Part model, mm, in its own coordinate system. Face numbers are marked on the shaded views. A direction names the side the tool comes from. Coordinates: 2 decimals unless noted, no trailing zeros. Loops run counter-clockwise (first coordinate to the right, second up) from the corner with the lowest first, then second, coordinate; pieces in that order, holes last. Notation, with made-up numbers: (-29, 59) -> (-6, 59) arc R28 ccw to (-6, 87) -> close; hole circle Ø11 at (75, 55). An arc over 180 degrees is marked (long way). One line per item, written item: value. Start each with the question number.
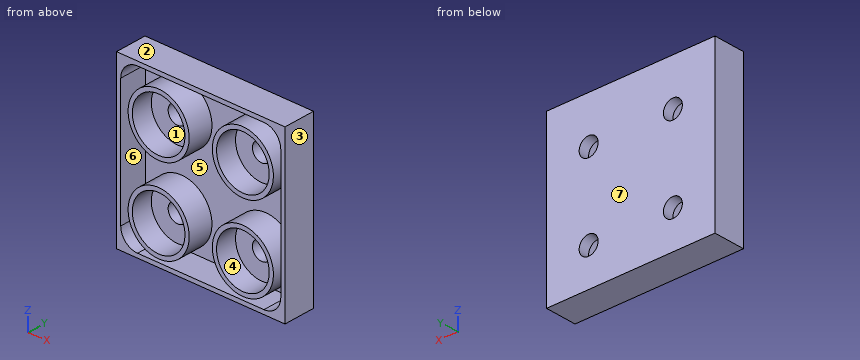
from build123d import *

# Parameters (mm, degrees)
CROQUIS1_W              = 40
CROQUIS1_H              = 40
CROQUIS1_R              = 2.25
SALIENTE_EXTRUIR1_DEPTH = 7.5
CROQUIS2_R              = 6.25
CORTAR_EXTRUIR1_DEPTH   = 5
VACIADO1_T              = -1
REDONDEO1_R             = 4


with BuildPart() as part:
    # Croquis1 → Saliente-Extruir1 (new body)
    with BuildSketch(Plane(origin=(0, 0, 0), x_dir=(1, 0, 0), z_dir=(0, 1, 0))):
        Rectangle(CROQUIS1_W, CROQUIS1_H)
        with Locations(Location((-10, -9, 0), (0, 0, 270))):
            Circle(CROQUIS1_R, mode=Mode.SUBTRACT)
        with Locations(Location((10, -9, 0), (0, 0, 270))):
            Circle(CROQUIS1_R, mode=Mode.SUBTRACT)
        with Locations(Location((10, 11, 0), (0, 0, 270))):
            Circle(CROQUIS1_R, mode=Mode.SUBTRACT)
        with Locations(Location((-10, 11, 0), (0, 0, 270))):
            Circle(CROQUIS1_R, mode=Mode.SUBTRACT)
    extrude(amount=SALIENTE_EXTRUIR1_DEPTH)

    # Croquis2 → Cortar-Extruir1 (cut)
    with BuildSketch(Plane.XZ):
        with Locations(Location((-10, 9, 0), (0, 0, 270))):
            Circle(CROQUIS2_R)
        with Locations(Location((10, 9, 0), (0, 0, 270))):
            Circle(CROQUIS2_R)
        with Locations(Location((-10, -11, 0), (0, 0, 270))):
            Circle(CROQUIS2_R)
        with Locations(Location((10, -11, 0), (0, 0, 270))):
            Circle(CROQUIS2_R)
    extrude(amount=-CORTAR_EXTRUIR1_DEPTH, mode=Mode.SUBTRACT)

    # Vaciado1
    vaciado1_openings = [part.faces().sort_by_distance(p)[0] for p in [
        (0, 0, 0.442577116),
    ]]
    offset(amount=VACIADO1_T, openings=vaciado1_openings, kind=Kind.INTERSECTION)

    # Redondeo1
    redondeo1_edges = [part.edges().sort_by_distance(p)[0] for p in [
        (-19, 3.25, -19),
        (19, 3.25, -19),
        (19, 3.25, 19),
        (-19, 3.25, 19),
    ]]
    fillet(redondeo1_edges, radius=REDONDEO1_R)


solid = part.part
1) Tool access for the marked faces 5, 6 and 7: list every direction of +Z, -Z, +X, -X, +Y, -Y with a clear straight run to the whole face (end or side of a thin tool).
2) Slice it at A-A (y = 3.5). State how many separate pieces and enclosed holes the cut face has, then the cut area to 3 significant figures.
3) Pull direction Z, two halves, no side cores. Call the marked faces 1, 2, 3 and 4: +Z half, -Z half, draft (parallel to the pull), parting line (faces both ways), or undercut.
4) Probe line 1 (X direction, y = 1.35, z = 9); line 2 (X direction, y = 3.5, z = -1); line 3 (X direction, y = 6.2, z = 9). List the from-to ranges inside material, lowest first. Write a range as from..to.
5) Slice it at B-B (z = -2.5). Give the cut face in (x, y), then the cut area to 3 significant figures.
6) Pin check, flat tips, straight feed: pin 1 Ø12 at (x, z) = (6, -15) entering from -Y; pin 2 Ø7 at (x, z) = (10, -11) entering from -Y. Stop position of each tip, or through.
Check sheet entries:
1. face 5: none
1. face 6: -Y
1. face 7: +Z, -Z, +X, -X, +Y
2. separate pieces: 5
2. enclosed holes: 5
2. area: 339 mm^2
3. face 1: undercut
3. face 2: +Z half
3. face 3: draft
3. face 4: undercut
4. line 1: x = -20..-19, -17.25..-16.25, -3.75..-2.75, 2.75..3.75, 16.25..17.25, 19..20
4. line 2: x = -20..-19, 19..20
4. line 3: x = -20..-19, -13.25..-12.25, -7.75..-6.75, 6.75..7.75, 12.25..13.25, 19..20
5. outline: (-20, 0) -> (-19, 0) -> (-19, 6.5) -> (19, 6.5) -> (19, 0) -> (20, 0) -> (20, 7.5) -> (-20, 7.5) -> close
5. area: 53.0 mm^2
6. pin 1: stops at y = 0
6. pin 2: stops at y = 5
